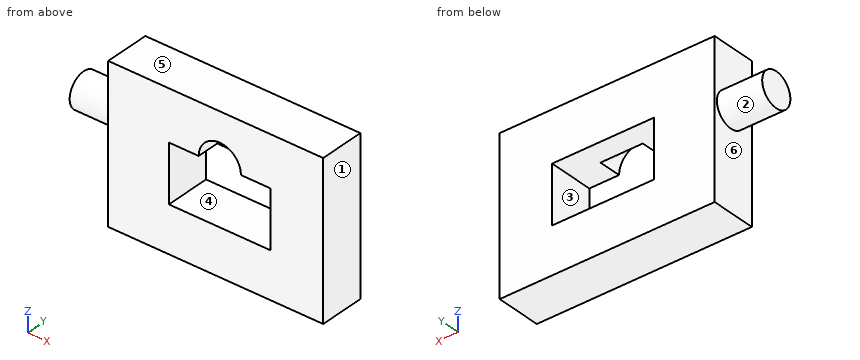
from build123d import *

# Parameters (mm, degrees)
F0_W     = 95
F0_H     = 67.8552658787
F0_W_2   = 44.9852889642
F0_H_2   = 25.2932771593
F1_DEPTH = 20
F2_R     = 7.5681331321
F3_DEPTH = 20
F5_DEPTH = 10


with BuildPart() as f1:
    # F0 (on Front) → F1 (new body)
    with BuildSketch(Plane.XZ):
        with Locations((-39.7814000025, 0.315669924)):
            Rectangle(F0_W, F0_H)
        with Locations((-37.9652246557, -0.5571056452)):
            Rectangle(F0_W_2, F0_H_2, mode=Mode.SUBTRACT)
    extrude(amount=F1_DEPTH)

    # F2 (on face) → F3 (join)
    with BuildSketch(Plane(origin=(-87.2814000025, 0, 0), x_dir=(0, -1, 0), z_dir=(-1, 0, 0))):
        with Locations((8.808799088, 8.3959847689)):
            Circle(F2_R)
    extrude(amount=F3_DEPTH)

    # F4 (on face) → F5 (cut)
    with BuildSketch(Plane.XZ.offset(20)):
        with BuildLine():
            Line((-47.3015092245, 12.0895329345), (-28.628940087, 12.0895329345))
            ThreePointArc((-28.628940087, 12.0895329345), (-37.9652246557, 21.4258175032), (-47.3015092245, 12.0895329345))
        make_face()
    extrude(amount=-F5_DEPTH, mode=Mode.SUBTRACT)


solid = f1.part
Design review of the part built by this model. Coordinates are the model's own, in mm. Face numbers are marked on the shaded views. A direction names the side the tool comes from. Coordinates: 2 decimals unless noted, no trailing zeros. Loops run counter-clockwise (first coordinate to the right, second up) from the corner with the lowest first, then second, coordinate; pieces in that order, holes last. Notation, with made-up numbers: M 66.5,-32 L 72.5,-32 A24 ccw 72.5,-9 Z; hole C 28,14 d2. An arc over 180 degrees is marked long. Answer as CSV lines item,"result".
Item 1: For P1, Ø4.5, axis at x = -36.5, z = 15, coming from the -Y side; P2, Ø5, axis at y = -16, z = -10.5, coming from the -X side, all flat-tipped, find the tip position at first contact; note any pin that passes through.
Answer list:
P1,"y = -10"
P2,"x = -87.28"
Item 2: For probe 1 along Z at (x, y) = (-45.5, -9.25); probe 2 along X at (y, z) = (-14.75, 10); probe 3 along X at (y, z) = (-17.5, 9.5), list the stretches that pass through material, from the lowest coordinate up.
Answer list:
probe 1,"-33.61 to -13.2, 12.09 to 34.24"
probe 2,"-107.28 to -60.46, -15.47 to 7.72"
probe 3,"-87.28 to -60.46, -15.47 to 7.72"
Item 3: Add section C-C on y = -3.75. State the section outline as (x, z) points, plus the area to 3 significant figures.
Answer list:
outline,"M -107.28,2.77 L -87.28,2.77 L -87.28,-33.61 L 7.72,-33.61 L 7.72,34.24 L -87.28,34.24 L -87.28,14.02 L -107.28,14.02 Z; hole M -60.46,-13.2 L -15.47,-13.2 L -15.47,12.09 L -60.46,12.09 Z"
area,"5,530 mm²"
Item 4: Machinability: for the marked faces 1, 2 and 3, which of the approach directions +Z, -Z, +X, -X, +Y, -Y give a long, thin tool a straight path to every point of the face, cutting with its end or side? Answer none if there is none.
Answer list:
face 1,"+Z, -Z, +X, +Y, -Y"
face 2,"-X"
face 3,"+Y, -Y"
Item 5: Add section D-D on z = -27.5. State the section outline as (x, y) points, plus the area to 3 significant figures.
Answer list:
outline,"M -87.28,-20 L 7.72,-20 L 7.72,0 L -87.28,0 Z"
area,"1,900 mm²"
Item 6: Add section B-B on x = -44. State the section outline as (y, z) points.
Answer list:
outline,"M -20,-33.61 L 0,-33.61 L 0,-13.2 L -20,-13.2 Z; M -20,19.21 L -10,19.21 L -10,12.09 L 0,12.09 L 0,34.24 L -20,34.24 Z"
Item 7: The part is to be moulded in two halves that separate along X. For the marked faces 4, 5 and 6, say which applies: pulls with the +X half, pulls with the -X half, needs draft (parallel to the pull), parting line crosses it, or undercut.
Answer list:
face 4,"undercut"
face 5,"needs draft"
face 6,"pulls with the -X half"
Item 8: Add section A-A on z = -3.5. State the section outline as (x, y) points, plus the area to 3 significant figures.
Answer list:
outline,"M -87.28,-20 L -60.46,-20 L -60.46,0 L -87.28,0 Z; M -15.47,-20 L 7.72,-20 L 7.72,0 L -15.47,0 Z"
area,"1,000 mm²"
